```python
from build123d import *

# Parameters (mm, degrees)
F1_DEPTH = 2


with BuildPart() as f1:
    # F0 (on Top) → F1 (new body)
    with BuildSketch(Plane.XY):
        Polygon((4, 25.754048), (0, 25.754048), (-4, 25.754048), (-7.5, -33.245952), (0, -33.245952), (7.5, -33.245952), align=None)
        Polygon((-4.089832, -29.330796), (-6.573987, -31.641873), (-6.292557, -27.084958), align=None, mode=Mode.SUBTRACT)
        Polygon((-6.13311, -24.568204), (-5.796553, -18.894804), (-3.715754, -21.609863), align=None, mode=Mode.SUBTRACT)
        Polygon((-1.067552, -32.354102), (-5.965223, -32.354102), (-3.397664, -29.978383), align=None, mode=Mode.SUBTRACT)
        Polygon((-3.404538, -28.675417), (-5.447618, -26.563399), (-1.229849, -26.563399), align=None, mode=Mode.SUBTRACT)
        Polygon((-0.45485, -31.733501), (-2.811431, -29.330796), (-0.45485, -27.101166), align=None, mode=Mode.SUBTRACT)
        Polygon((-5.633629, -25.496741), (-3.286195, -22.381087), (-0.96125, -25.496741), align=None, mode=Mode.SUBTRACT)
        Polygon((-3.17182, -20.85387), (-5.191417, -18.046699), (-0.996083, -18.046699), align=None, mode=Mode.SUBTRACT)
        Polygon((-2.601866, -21.61763), (-0.45485, -18.894804), (-0.45485, -24.601909), align=None, mode=Mode.SUBTRACT)
        Polygon((-3.465, -12.372064), (-5.633629, -15.68081), (-5.260959, -9.398653), align=None, mode=Mode.SUBTRACT)
        Polygon((-0.799204, -16.985185), (-5.30343, -16.985185), (-2.959617, -13.249483), align=None, mode=Mode.SUBTRACT)
        Polygon((-2.357842, -12.361948), (-0.45485, -9.398653), (-0.45485, -15.858355), align=None, mode=Mode.SUBTRACT)
        Polygon((-2.892819, -11.457191), (-4.714794, -8.298798), (-0.8917, -8.298798), align=None, mode=Mode.SUBTRACT)
        Polygon((-0.799204, -7.197334), (-4.789895, -7.197334), (-2.633869, -3.756868), align=None, mode=Mode.SUBTRACT)
        Polygon((2.811431, -29.330796), (0.45485, -31.733501), (0.45485, -27.101166), align=None, mode=Mode.SUBTRACT)
        Polygon((5.965223, -32.354102), (1.067552, -32.354102), (3.397664, -29.978383), align=None, mode=Mode.SUBTRACT)
        Polygon((5.447618, -26.563399), (3.404538, -28.675417), (1.229849, -26.563399), align=None, mode=Mode.SUBTRACT)
        Polygon((0.45485, -18.894804), (2.601866, -21.61763), (0.45485, -24.601909), align=None, mode=Mode.SUBTRACT)
        Polygon((3.286195, -22.381087), (5.633629, -25.496741), (0.96125, -25.496741), align=None, mode=Mode.SUBTRACT)
        Polygon((0.996083, -18.046699), (5.191417, -18.046699), (3.17182, -20.85387), align=None, mode=Mode.SUBTRACT)
        Polygon((6.292557, -27.084958), (6.573987, -31.641873), (4.089832, -29.330796), align=None, mode=Mode.SUBTRACT)
        Polygon((5.796553, -18.894804), (6.13311, -24.568204), (3.715754, -21.609863), align=None, mode=Mode.SUBTRACT)
        Polygon((2.357842, -12.361948), (0.45485, -15.858355), (0.45485, -9.398653), align=None, mode=Mode.SUBTRACT)
        Polygon((0.799204, -16.985185), (2.959617, -13.249483), (5.30343, -16.985185), align=None, mode=Mode.SUBTRACT)
        Polygon((0.8917, -8.298798), (4.714794, -8.298798), (2.892819, -11.457191), align=None, mode=Mode.SUBTRACT)
        Polygon((4.789895, -7.197334), (0.799204, -7.197334), (2.633869, -3.756868), align=None, mode=Mode.SUBTRACT)
        Polygon((3.465, -12.372064), (5.260959, -9.398653), (5.633629, -15.68081), align=None, mode=Mode.SUBTRACT)
        Polygon((-5.060531, -5.828136), (-4.714794, 0), (-3.17182, -2.843706), align=None, mode=Mode.SUBTRACT)
        Polygon((-2.611527, -1.832106), (-4.170251, 1.077535), (-0.799204, 1.077535), align=None, mode=Mode.SUBTRACT)
        Polygon((-2.009785, -2.843706), (-0.45485, -0.113241), (-0.45485, -5.948542), align=None, mode=Mode.SUBTRACT)
        Polygon((-4.450015, 3.616143), (-4.170251, 8.613745), (-2.811431, 6.248467), align=None, mode=Mode.SUBTRACT)
        Polygon((-0.799204, 2.134794), (-4.170251, 2.134794), (-2.357842, 5.247023), align=None, mode=Mode.SUBTRACT)
        Polygon((-2.271924, 7.201679), (-3.641225, 9.758234), (-0.799204, 9.758234), align=None, mode=Mode.SUBTRACT)
        Polygon((-1.841009, 6.179651), (-0.45485, 8.613745), (-0.45485, 3.411822), align=None, mode=Mode.SUBTRACT)
        Polygon((-3.910219, 12.291129), (-3.715754, 16.559127), (-2.614767, 14.565943), align=None, mode=Mode.SUBTRACT)
        Polygon((-0.799204, 10.940004), (-3.641225, 10.940004), (-2.120922, 13.579161), align=None, mode=Mode.SUBTRACT)
        Polygon((-2.069376, 15.469204), (-3.286195, 17.699626), (-0.799204, 17.699626), align=None, mode=Mode.SUBTRACT)
        Polygon((-0.45485, 12.224307), (-1.568874, 14.448747), (-0.45485, 16.402385), align=None, mode=Mode.SUBTRACT)
        Polygon((-0.661599, 18.764926), (-3.286195, 18.764926), (-1.841009, 21.210955), align=None, mode=Mode.SUBTRACT)
        Polygon((-3.465, 20.303925), (-3.286195, 23.963032), (-2.357842, 22.213539), align=None, mode=Mode.SUBTRACT)
        Polygon((-1.841009, 23.178602), (-2.811431, 25.27616), (-0.76812, 25.27616), align=None, mode=Mode.SUBTRACT)
        Polygon((-1.39996, 22.213539), (-0.45485, 23.963032), (-0.429307, 20.278619), align=None, mode=Mode.SUBTRACT)
        Polygon((0.45485, -5.948542), (0.45485, -0.113241), (2.009785, -2.843706), align=None, mode=Mode.SUBTRACT)
        Polygon((0.799204, 1.077535), (4.170251, 1.077535), (2.611527, -1.832106), align=None, mode=Mode.SUBTRACT)
        Polygon((0.45485, 8.613745), (1.841009, 6.179651), (0.45485, 3.411822), align=None, mode=Mode.SUBTRACT)
        Polygon((0.799204, 2.134794), (2.357842, 5.247023), (4.170251, 2.134794), align=None, mode=Mode.SUBTRACT)
        Polygon((2.811431, 6.248467), (4.170251, 8.613745), (4.450015, 3.616143), align=None, mode=Mode.SUBTRACT)
        Polygon((2.271924, 7.201679), (0.799204, 9.758234), (3.641225, 9.758234), align=None, mode=Mode.SUBTRACT)
        Polygon((4.714794, 0), (5.060531, -5.828136), (3.17182, -2.843706), align=None, mode=Mode.SUBTRACT)
        Polygon((1.568874, 14.448747), (0.45485, 12.224307), (0.45485, 16.402385), align=None, mode=Mode.SUBTRACT)
        Polygon((0.799204, 10.940004), (2.120922, 13.579161), (3.641225, 10.940004), align=None, mode=Mode.SUBTRACT)
        Polygon((3.910219, 12.291129), (2.614767, 14.565943), (3.715754, 16.559127), align=None, mode=Mode.SUBTRACT)
        Polygon((0.799204, 17.699626), (3.286195, 17.699626), (2.069376, 15.469204), align=None, mode=Mode.SUBTRACT)
        Polygon((0.45485, 23.963032), (1.39996, 22.213539), (0.429307, 20.278619), align=None, mode=Mode.SUBTRACT)
        Polygon((0.76812, 25.27616), (2.811431, 25.27616), (1.841009, 23.178602), align=None, mode=Mode.SUBTRACT)
        Polygon((0.661599, 18.764926), (1.841009, 21.210955), (3.286195, 18.764926), align=None, mode=Mode.SUBTRACT)
        Polygon((3.465, 20.303925), (2.357842, 22.213539), (3.286195, 23.963032), align=None, mode=Mode.SUBTRACT)
    extrude(amount=F1_DEPTH)


solid = f1.part
```
Geometry check sheet. Reference: the model listing, model coordinates, mm. Coordinates: 2 decimals unless noted, no trailing zeros. One line per item, written item: value. Start each with the question number.
(1) Sectioned sample at A-A, the plane z = 0.6. State how many separate pieces and enclosed holes the cut face has, and give its area (3 significant figures).
(2) Release check for a two-part mould opening along X. For faces 1 (the face through (0, -3, 2)), 2 (the face through (1.543, -23.089, 0.986)) record: released by +X, released by -X, zero draft, split by the parting line, or undercut.
(3) Depth check by flat-ended pin: pin 1 (1 mm diameter, centred on y = 2, z = 1.5, fed in from +X); pin 2 (1 mm diameter, centred on y = -11, z = 1, fed in from -X). Enter the tip coordinate at first touch or a pass-through.
(4) Scan lines: line 1 along X through (y, z) = (11, 0.5); line 2 along X through (y, z) = (-27, 0.9); line 3 along X through (y, z) = (21.5, 1.55). Record each from-to range of solid material in increasing order. Write a range as [from, to].
Filled sheet:
1. separate pieces: 1
1. enclosed holes: 56
1. area: 416 mm²
2. face 1: zero draft
2. face 2: undercut
3. pin 1: x = 5.44
3. pin 2: x = -6.21
4. line 1: [-4.88, -3.61], [-0.83, 0.83], [3.61, 4.88]
4. line 2: [-7.13, -5.03], [-1.68, 1.68], [5.03, 7.13]
4. line 3: [-4.25, -3.41], [-2.77, -1.04], [-0.44, 0.44], [1.04, 2.77], [3.41, 4.25]
